from build123d import *

# Parameters (mm, degrees)
EXTRUDE_1_DEPTH    = 620
HOLE_WIZARD_M5_1_D = 4.2
FILLET_1_R         = 1
FILLET_2_R         = 0.5


with BuildPart() as part:
    # 草图1 → 凸台-拉伸1 (new body)
    with BuildSketch(Plane.XY):
        Polygon((0, 0), (0, 18), (-2.5, 18), (-2.5, 2), (-7.5, 2), (-7.5, 0), align=None)
    extrude(amount=EXTRUDE_1_DEPTH)

    # M5 螺纹孔1 (through all)
    with Locations(Plane(origin=(0, 0, 0), x_dir=(0, 0, -1), z_dir=(1, 0, 0))):
        with Locations((-496, 10), (-372, 10), (-248, 10), (-124, 10)):
            Hole(HOLE_WIZARD_M5_1_D / 2)

    # 圆角1
    fillet_1_edges = [part.edges().sort_by_distance(p)[0] for p in [
        (-2.5, 2, 310),
        (0, 0, 310),
    ]]
    fillet(fillet_1_edges, radius=FILLET_1_R)

    # 圆角2
    fillet_2_edges = [part.edges().sort_by_distance(p)[0] for p in [
        (-7.5, 0, 310),
        (-7.5, 2, 310),
        (-2.5, 18, 310),
        (0, 18, 310),
    ]]
    fillet(fillet_2_edges, radius=FILLET_2_R)


solid = part.part
Build history of the part. All positions in model axes, mm. A direction names the side the tool comes from. Coordinates: 2 decimals unless noted, no trailing zeros. Order: outer loops, then holes, each group sorted by start corner. A loop starts at its lowest first (then second) coordinate and runs counter-clockwise, first axis right, second up. Notation, with made-up numbers: (-39.75, -4.75) - (-7.75, -4.75) arc R26 ccw to (-7.75, 24.25) - close; hole circle Ø3 at (65, 58). An arc over 180 degrees is marked (long way). Put each result on its own line as item: value.
1. Saw through at A-A (z = 397). Write the cut outline in (x, y).
Answer sheet:
outline: (-7.5, 0.5) arc R0.5 ccw to (-7, 0) - (-1, 0) arc R1 ccw to (0, 1) - (0, 17.5) arc R0.5 ccw to (-0.5, 18) - (-2, 18) arc R0.5 ccw to (-2.5, 17.5) - (-2.5, 3) arc R1 cw to (-3.5, 2) - (-7, 2) arc R0.5 ccw to (-7.5, 1.5) - close
2. Drop flat-ended pins along their axis: P1, Ø3, axis at y = 4, z = 515.5, coming from the -X side; P2, Ø5, axis at y = 10, z = 496, coming from the +X side; P3, Ø5, axis at y = 10, z = 124, coming from the -X side; P4, Ø1.8, axis at x = -5, z = 317, coming from the +Y side. Give the stop position or say it passes through.
Answer sheet:
P1: stops at x = -2.63
P2: stops at x = 0
P3: stops at x = -2.5
P4: stops at y = 2
3. Tool access for faces 1 (the face through (-2.5, 10, 306)), 2 (the face through (0, 9, 306)): list every direction of +Z, -Z, +X, -X, +Y, -Y with a clear straight run to the whole face (end or side of a thin tool).
Answer sheet:
face 1: +Z, -Z, -X, +Y
face 2: +Z, -Z, +X, +Y, -Y
4. Saw through at B-B (x = -5.75). Write the cut outline in (y, z).
Answer sheet:
outline: (0, 0) - (2, 0) - (2, 620) - (0, 620) - close
5. Probe line 1 along Y through (x, z) = (-1.65, 248); line 2 along Y through (x, z) = (-0.6, 496); line 3 along Y through (x, z) = (-5.25, 520.5). List the from-to ranges inside material, lowest first. Write a range as [from, to].
Answer sheet:
line 1: y = [0, 7.9], [12.1, 18]
line 2: y = [0.08, 7.9], [12.1, 18]
line 3: y = [0, 2]
